Autodesk Inventor part; units mm, degrees
ref_plane "YZ Plane" through (0, 0, 0) normal (1, 0, 0) x (0, 1, 0)
ref_plane "XZ Plane" through (0, 0, 0) normal (0, 1, 0) x (-1, 0, 0)
ref_plane "XY Plane" through (0, 0, 0) normal (0, 0, 1) x (1, 0, 0)
sketch "Sketch1" plane through (0, 0, 0) normal (0, 1, 0) x (-1, 0, 0)
  circle A0 centre (0, 0) radius 16
  circle A1 centre (8, -8) radius 2.1
  circle A2 centre (8, 8) radius 2.1
  circle A3 centre (-8, 8) radius 2.1
  circle A4 centre (-8, -8) radius 2.1
  dimension "d0" = 32
  dimension "d1" = 4.2
  dimension "d2" = 8
  dimension "d3" = 8
  dimension "d6" = 360
extrude "Extrusion1" add sketch "Sketch1" along normal blind 3
properties part number "WristSpaacer"
The listing builds one solid part. Answer for the finished solid, in the listing's coordinates (mm). Round coordinates to 2 decimals unless told otherwise and drop trailing zeros. Order: outer loops, then holes, each group sorted by start corner. A loop starts at its lowest first (then second) coordinate and runs counter-clockwise, first axis right, second up. Notation, with made-up numbers: (14.25, 87) -> (60.25, 87) arc R13 ccw to (60.25, 96) -> close; hole circle Ø7 at (84.5, 52.5). An arc over 180 degrees is marked (long way). Answer as CSV lines item,"result".
Q1. Consider line 1 (Z direction, x = -8, y = 1.05); line 2 (X direction, y = 0.55, z = 7); line 3 (X direction, y = 2.1, z = -2). Determine where each line is inside the solid, lowest interval first. Write a range as from..to.
Computed values:
line 1,"z = -13.86..-10.1, -5.9..5.9, 10.1..13.86"
line 2,"x = -14.39..-9.85, -6.15..6.15, 9.85..14.39"
line 3,"x = -15.87..15.87"
Q2. Given pin 1 (4 mm diameter, centred on x = 8, z = -8, fed in from +Y); pin 2 (1.5 mm diameter, centred on y = 1, z = 6.5, fed in from +X), each flat-ended and moving along its own axis, determine where each tip first touches the part or whether it passes through.
Computed values:
pin 1,"passes through"
pin 2,"stops at x = 14.93"
Q3. A cutting plane is placed at C-C on y = 1.95. Determine the outline of the cut face in (x, z).
Computed values:
outline,"circle Ø32 at (0, 0); hole circle Ø4.2 at (-8, -8); hole circle Ø4.2 at (-8, 8); hole circle Ø4.2 at (8, -8); hole circle Ø4.2 at (8, 8)"
Q4. A cutting plane is placed at B-B on x = 7.5. Determine the outline of the cut face in (y, z).
Computed values:
outline,"(0, -14.13) -> (3, -14.13) -> (3, -10.04) -> (0, -10.04) -> close; (0, -5.96) -> (3, -5.96) -> (3, 5.96) -> (0, 5.96) -> close; (0, 10.04) -> (3, 10.04) -> (3, 14.13) -> (0, 14.13) -> close"
Q5. A cutting plane is placed at A-A on z = -8. Determine the outline of the cut face in (x, y), plus the area to 3 significant figures.
Computed values:
outline,"(-13.86, 0) -> (-10.1, 0) -> (-10.1, 3) -> (-13.86, 3) -> close; (-5.9, 0) -> (5.9, 0) -> (5.9, 3) -> (-5.9, 3) -> close; (10.1, 0) -> (13.86, 0) -> (13.86, 3) -> (10.1, 3) -> close"
area,"57.9 mm^2"
Q6. A cutting plane is placed at D-D on z = 11. Determine the outline of the cut face in (x, y), plus the area to 3 significant figures.
Computed values:
outline,"(-11.62, 0) -> (11.62, 0) -> (11.62, 3) -> (-11.62, 3) -> close"
area,"69.7 mm^2"
Q7. For a pull along X with two mould halves and no side action, classify faces 1 (the cylindrical face through (3.47, 1.48, 15.62)), 2 (the flat face through (0, 0, 0)), 3 (the cylindrical face through (8.273, 1.479, -10.082)) as +X half, -X half, draft (parallel to the pull), parting line (faces both ways), or undercut.
Computed values:
face 1,"parting line"
face 2,"draft"
face 3,"undercut"
